Model file for the job. Use its own axes, mm. A direction names the side the tool comes from. Give positions to 0.01 mm unless a question says otherwise; leave off trailing zeros. Answer in a Markdown table with one row per item.
```python
from build123d import *

# Parameters (mm, degrees)
SKETCH_1_R      = 3.4
SKETCH_1_R_2    = 4.3
EXTRUDE_1_DEPTH = 1000


with BuildPart() as part:
    # Эскиз1 → Бобышка-Вытянуть1 (new body)
    with BuildSketch(Plane.XY):
        with BuildLine():
            Line((-20, 47.3), (-20, 60))
            Line((-20, 60), (-7.3, 60))
            Line((-7.3, 60), (-4.2, 60))
            Line((-4.2, 60), (-4.2, 56.4))
            Line((-4.2, 56.4), (-7.3, 56.4))
            Line((-7.3, 56.4), (-7.3, 49.4))
            ThreePointArc((-7.3, 49.4), (0, 45.979473661), (7.3, 49.4))
            Line((7.3, 49.4), (7.3, 56.4))
            Line((7.3, 56.4), (4.2, 56.4))
            Line((4.2, 56.4), (4.2, 60))
            Line((4.2, 60), (7.3, 60))
            Line((7.3, 60), (20, 60))
            Line((20, 60), (20, 47.3))
            Line((20, 47.3), (20, 44.2))
            Line((20, 44.2), (16.4, 44.2))
            Line((16.4, 44.2), (16.4, 47.3))
            Line((16.4, 47.3), (9.4, 47.3))
            ThreePointArc((9.4, 47.3), (5.979473661, 40), (9.4, 32.7))
            Line((9.4, 32.7), (16.4, 32.7))
            Line((16.4, 32.7), (16.4, 35.8))
            Line((16.4, 35.8), (20, 35.8))
            Line((20, 35.8), (20, 32.7))
            Line((20, 32.7), (20, 29))
            ThreePointArc((20, 29), (13.636038969, 13.636038969), (29, 20))
            Line((29, 20), (32.7, 20))
            Line((32.7, 20), (35.8, 20))
            Line((35.8, 20), (35.8, 16.4))
            Line((35.8, 16.4), (32.7, 16.4))
            Line((32.7, 16.4), (32.7, 9.4))
            ThreePointArc((32.7, 9.4), (40, 5.979473661), (47.3, 9.4))
            Line((47.3, 9.4), (47.3, 16.4))
            Line((47.3, 16.4), (44.2, 16.4))
            Line((44.2, 16.4), (44.2, 20))
            Line((44.2, 20), (47.3, 20))
            Line((47.3, 20), (60, 20))
            Line((60, 20), (60, 7.3))
            Line((60, 7.3), (60, 4.2))
            Line((60, 4.2), (56.4, 4.2))
            Line((56.4, 4.2), (56.4, 7.3))
            Line((56.4, 7.3), (49.4, 7.3))
            ThreePointArc((49.4, 7.3), (45.979473661, 0), (49.4, -7.3))
            Line((49.4, -7.3), (56.4, -7.3))
            Line((56.4, -7.3), (56.4, -4.2))
            Line((56.4, -4.2), (60, -4.2))
            Line((60, -4.2), (60, -7.3))
            Line((60, -7.3), (60, -20))
            Line((60, -20), (47.3, -20))
            Line((47.3, -20), (44.2, -20))
            Line((44.2, -20), (44.2, -16.4))
            Line((44.2, -16.4), (47.3, -16.4))
            Line((47.3, -16.4), (47.3, -9.4))
            ThreePointArc((47.3, -9.4), (40, -5.979473661), (32.7, -9.4))
            Line((32.7, -9.4), (32.7, -16.4))
            Line((32.7, -16.4), (35.8, -16.4))
            Line((35.8, -16.4), (35.8, -20))
            Line((35.8, -20), (32.7, -20))
            Line((32.7, -20), (7.3, -20))
            Line((7.3, -20), (4.2, -20))
            Line((4.2, -20), (4.2, -16.4))
            Line((4.2, -16.4), (7.3, -16.4))
            Line((7.3, -16.4), (7.3, -9.4))
            ThreePointArc((7.3, -9.4), (0, -5.979473661), (-7.3, -9.4))
            Line((-7.3, -9.4), (-7.3, -16.4))
            Line((-7.3, -16.4), (-4.2, -16.4))
            Line((-4.2, -16.4), (-4.2, -20))
            Line((-4.2, -20), (-7.3, -20))
            Line((-7.3, -20), (-20, -20))
            Line((-20, -20), (-20, -7.3))
            Line((-20, -7.3), (-20, -4.2))
            Line((-20, -4.2), (-16.4, -4.2))
            Line((-16.4, -4.2), (-16.4, -7.3))
            Line((-16.4, -7.3), (-9.4, -7.3))
            ThreePointArc((-9.4, -7.3), (-5.979473661, 0), (-9.4, 7.3))
            Line((-9.4, 7.3), (-16.4, 7.3))
            Line((-16.4, 7.3), (-16.4, 4.2))
            Line((-16.4, 4.2), (-20, 4.2))
            Line((-20, 4.2), (-20, 7.3))
            Line((-20, 7.3), (-20, 32.7))
            Line((-20, 32.7), (-20, 35.8))
            Line((-20, 35.8), (-16.4, 35.8))
            Line((-16.4, 35.8), (-16.4, 32.7))
            Line((-16.4, 32.7), (-9.4, 32.7))
            ThreePointArc((-9.4, 32.7), (-5.979473661, 40), (-9.4, 47.3))
            Line((-9.4, 47.3), (-16.4, 47.3))
            Line((-16.4, 47.3), (-16.4, 44.2))
            Line((-16.4, 44.2), (-20, 44.2))
            Line((-20, 44.2), (-20, 47.3))
        make_face()
        with Locations((0, 40)):
            Circle(SKETCH_1_R, mode=Mode.SUBTRACT)
        with Locations((-13.5, 53.5)):
            Circle(SKETCH_1_R_2, mode=Mode.SUBTRACT)
        with Locations((13.5, 53.5)):
            Circle(SKETCH_1_R_2, mode=Mode.SUBTRACT)
        with Locations((-13.5, -13.5)):
            Circle(SKETCH_1_R_2, mode=Mode.SUBTRACT)
        Circle(SKETCH_1_R, mode=Mode.SUBTRACT)
        with Locations((40, 0)):
            Circle(SKETCH_1_R, mode=Mode.SUBTRACT)
        with Locations((53.5, 13.5)):
            Circle(SKETCH_1_R_2, mode=Mode.SUBTRACT)
        with Locations((53.5, -13.5)):
            Circle(SKETCH_1_R_2, mode=Mode.SUBTRACT)
        with BuildLine():
            Line((-2.207961827, 4.707961827), (-7.5, 10))
            Line((-7.5, 10), (-18, 10))
            Line((-18, 10), (-18, 30))
            Line((-18, 30), (-9, 30))
            Line((-9, 30), (-5.450961894, 32.049038106))
            Line((-5.450961894, 32.049038106), (-3.5, 34))
            Line((-3.5, 34), (3.5, 34))
            Line((3.5, 34), (5.450961894, 32.049038106))
            Line((5.450961894, 32.049038106), (9, 30))
            Line((9, 30), (14.737871153, 30))
            ThreePointArc((14.737871153, 30), (12.009693373, 12.009693373), (30, 14.737871153))
            Line((30, 14.737871153), (30, 9))
            Line((30, 9), (32.049038106, 5.450961894))
            Line((32.049038106, 5.450961894), (34, 3.5))
            Line((34, 3.5), (34, -3.5))
            Line((34, -3.5), (32.049038106, -5.450961894))
            Line((32.049038106, -5.450961894), (30, -9))
            Line((30, -9), (30, -18))
            Line((30, -18), (10, -18))
            Line((10, -18), (10, -7.5))
            Line((10, -7.5), (4.707961827, -2.207961827))
            ThreePointArc((4.707961827, -2.207961827), (3.676955262, 3.676955262), (-2.207961827, 4.707961827))
        make_face(mode=Mode.SUBTRACT)
    extrude(amount=EXTRUDE_1_DEPTH)


solid = part.part
```
Q1. Mould opens along Y. For faces 4 (the face through (-18, 20, 493)), 5 (the face through (60, 12, 493)), 6 (the face through (-12, 60, 493)) say: released by +Y, released by -Y, zero draft, split by the parting line, or undercut.
Reported:
| item | result |
|---|---|
| face 4 | undercut |
| face 5 | zero draft |
| face 6 | released by +Y |
Q2. Saw through at A-A (z = 712). Give the number of separate pieces and of enclosed holes in the cut face, and give its area (3 significant figures).
Reported:
| item | result |
|---|---|
| separate pieces | 1 |
| enclosed holes | 9 |
| area | 1,520 mm² |
Q3. Probe probe 1 along Y at (x, z) = (1, 820); probe 2 along X at (y, z) = (0.5, 420); probe 3 along Y at (x, z) = (53.5, 397.5). List the from-to ranges inside material, lowest first.
Reported:
| item | result |
|---|---|
| probe 1 | -6.03 to -3.25, 3.25 to 5.1, 34 to 36.75, 43.25 to 46.03 |
| probe 2 | -5.99 to -3.36, 3.36 to 5.18, 34 to 36.64, 43.36 to 45.99 |
| probe 3 | -20 to -17.8, -9.2 to -7.3, 7.3 to 9.2, 17.8 to 20 |
Q4. Drop flat-ended pins along their axis: pin 1 (2 mm diameter, centred on y = 43, z = 371, fed in from -X); pin 2 (1 mm diameter, centred on y = 38, z = 681, fed in from +X); pin 3 (3 mm diameter, centred on x = 40.5, z = 805.5, fed in from -Y); pin 4 (10 mm diameter, centred on x = 53.5, y = 13.5, fed in from -Z). Give the stop position or say it passes through.
Reported:
| item | result |
|---|---|
| pin 1 | x = -6.86 |
| pin 2 | x = 6.31 |
| pin 3 | y = -6.19 |
| pin 4 | z = 0 |
Q5. 3-axis set-ups, long thin cutter, end or side, ignore diameter. For faces 1 (the face through (20, 52, 493)), 2 (the face through (60, -12, 493)), 3 (the face through (20, -18, 493)): which of +Z, -Z, +X, -X, +Y, -Y reach the whole face in a straight line?
Reported:
| item | result |
|---|---|
| face 1 | +Z, -Z, +X, +Y |
| face 2 | +Z, -Z, +X, +Y, -Y |
| face 3 | +Z, -Z |
